Source: CAD feature listing. Evaluate the final solid. Frame: model axes, mm. A direction names the side the tool comes from. Coordinates: 2 decimals unless noted, no trailing zeros. Loops run counter-clockwise (first coordinate to the right, second up) from the corner with the lowest first, then second, coordinate; pieces in that order, holes last. Notation, with made-up numbers: (73.5, 72.5) -> (87.5, 72.5) arc R16 cw to (87.5, 92.5) -> close; hole circle Ø11 at (73.5, 88). An arc over 180 degrees is marked (long way). Answer as CSV lines item,"result".
from build123d import *

# Parameters (mm, degrees)
SKETCH_R        = 7.5
PAD_DEPTH       = 8
SKETCH001_R     = 4.5
PAD001_DEPTH    = 21
SKETCH002_R     = 6.5
SKETCH002_R_2   = 5.5
POCKET_DEPTH    = 2
SKETCH003_R     = 3
POCKET001_DEPTH = 25
POCKET002_DEPTH = 5


with BuildPart() as part:
    # Sketch → Pad (new body)
    with BuildSketch(Plane.XY):
        Circle(SKETCH_R)
    extrude(amount=PAD_DEPTH)

    # Sketch001 (on Face3 of Pad) → Pad001 (join)
    with BuildSketch(Plane.XY.offset(8)):
        Circle(SKETCH001_R)
    extrude(amount=PAD001_DEPTH)

    # Sketch002 (on Face3 of Pad001) → Pocket (cut)
    with BuildSketch(Plane.XY.offset(8)):
        Circle(SKETCH002_R)
        Circle(SKETCH002_R_2, mode=Mode.SUBTRACT)
    extrude(amount=-POCKET_DEPTH, mode=Mode.SUBTRACT)

    # Sketch003 (on Face9 of Pocket) → Pocket001 (cut)
    with BuildSketch(Plane.XY.offset(29)):
        Circle(SKETCH003_R)
    extrude(amount=-POCKET001_DEPTH, mode=Mode.SUBTRACT)

    # Sketch004 (on Face2 of Pocket001) → Pocket002 (cut)
    with BuildSketch(Plane(origin=(0, 0, 0), x_dir=(1, 0, 0), z_dir=(0, 0, -1))):
        Polygon((3.660254, -3.660254), (5, 1.339746), (1.339746, 5), (-3.660254, 3.660254), (-5, -1.339746), (-1.339746, -5), align=None)
    extrude(amount=-POCKET002_DEPTH, mode=Mode.SUBTRACT)


solid = part.part
(1) Material intervals for L1, parallel to Y at x = 0, z = 7.45; L2, parallel to Y at x = 0, z = 17; L3, parallel to X at y = -0.5, z = 27.5, sorted ascending. Write a range as [from, to].
Computed values:
L1,"[-7.5, -6.5], [-5.5, -3], [3, 5.5], [6.5, 7.5]"
L2,"[-4.5, -3], [3, 4.5]"
L3,"[-4.47, -2.96], [2.96, 4.47]"
(2) Cut plane B-B (z = 6.75). Return the cut outline in (x, y).
Computed values:
outline,"circle Ø15 at (0, 0); circle Ø11 at (0, 0); hole circle Ø13 at (0, 0); hole circle Ø6 at (0, 0)"
(3) Pin query (flat end, axial travel): pin 1 Ø1 at (x, z) = (-2.5, 3) entering from -Y; pin 2 Ø8 at (y, z) = (1, 25) entering from -X; pin 3 Ø1 at (x, z) = (2, 10) entering from +Y. Return the tip coordinate at first contact, or that it passes through.
Computed values:
pin 1,"y = -7.23"
pin 2,"x = -4.5"
pin 3,"y = 4.24"
(4) Cut plane A-A (z = 3.75). Return the cut outline in (x, y), then the cut area to 3 significant figures.
Computed values:
outline,"circle Ø15 at (0, 0); hole (-5, 1.34) -> (-3.66, -3.66) -> (1.34, -5) -> (5, -1.34) -> (3.66, 3.66) -> (-1.34, 5) -> close"
area,"107 mm^2"
(5) Access query for faces 1 (the cylindrical face through (-1.19, -5.37, 7.01)), 2 (the flat face through (-4.32, -1.2, 2.46)), 3 (the flat face through (1, -3, 29)). Directions: +Z, -Z, +X, -X, +Y, -Y. A direction counts if a zero-diameter tool reaches every point of the face in a straight line with its end or side. Return the directions, or none.
Computed values:
face 1,"+Z"
face 2,"-Z"
face 3,"+Z, +X, -X, +Y, -Y"
(6) Draft query along Y for faces 4 (the flat face through (2.2, -2.3, 5)), 5 (the flat face through (-6, 3, 8)), 6 (the cylindrical face through (-0.59, 4.46, 18.35)). Return one class per face: released by +Y, released by -Y, zero draft, split by the parting line, or undercut.
Computed values:
face 4,"undercut"
face 5,"zero draft"
face 6,"split by the parting line"
(7) Cut plane C-C (x = 2.25). Return the cut outline in (y, z), then the cut area to 3 significant figures.
Computed values:
outline,"(-7.15, 0) -> (-4.09, 0) -> (-4.09, 5) -> (-1.98, 5) -> (-1.98, 29) -> (-3.9, 29) -> (-3.9, 8) -> (-5.02, 8) -> (-5.02, 6) -> (-6.1, 6) -> (-6.1, 8) -> (-7.15, 8) -> close; (1.98, 5) -> (4.04, 5) -> (4.04, 0) -> (7.15, 0) -> (7.15, 8) -> (6.1, 8) -> (6.1, 6) -> (5.02, 6) -> (5.02, 8) -> (3.9, 8) -> (3.9, 29) -> (1.98, 29) -> close"
area,"138 mm^2"
(8) Cut plane D-D (y = 0). Return the cut outline in (x, z).
Computed values:
outline,"(-7.5, 0) -> (-4.64, 0) -> (-4.64, 5) -> (-3, 5) -> (-3, 29) -> (-4.5, 29) -> (-4.5, 8) -> (-5.5, 8) -> (-5.5, 6) -> (-6.5, 6) -> (-6.5, 8) -> (-7.5, 8) -> close; (3, 5) -> (4.64, 5) -> (4.64, 0) -> (7.5, 0) -> (7.5, 8) -> (6.5, 8) -> (6.5, 6) -> (5.5, 6) -> (5.5, 8) -> (4.5, 8) -> (4.5, 29) -> (3, 29) -> close"
